The listing builds one solid part. Answer for the finished solid, in the listing's coordinates (mm). Face numbers are marked on the shaded views. Round coordinates to 2 decimals unless told otherwise and drop trailing zeros. Write each loop counter-clockwise with the first axis right and the second up, starting at its lowest first coordinate (ties: lowest second). Pieces come first, ordered by that corner, then holes. Notation, with made-up numbers: M -26,52.25 L 2,52.25 A21 ccw 2,83.25 Z; hole C 79.5,34.5 d3. An arc over 180 degrees is marked long. Write each question's results on one line, items separated by ' | '.
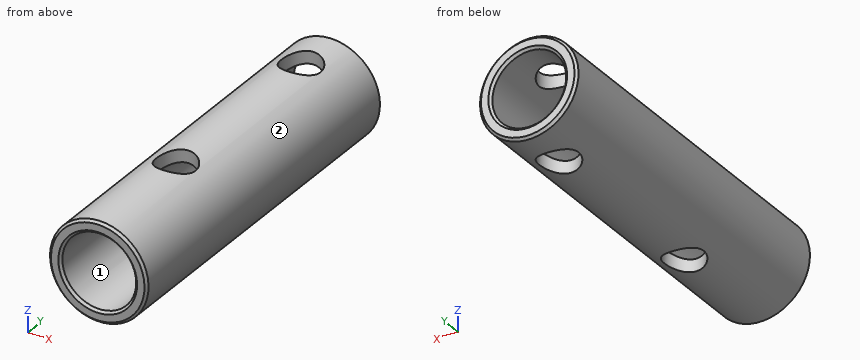
from build123d import *

# Parameters (mm, degrees)
SKIZZE1_R                       = 4
SKIZZE1_R_2                     = 3
AUFSATZ_LINEAR_AUSTRAGEN1_DEPTH = 30
FASE1_SIZE                      = 0.2
SKIZZE2_R                       = 1.6
SCHNITT_LINEAR_AUSTRAGEN1_DEPTH = 6


with BuildPart() as part:
    # Skizze1 → Aufsatz-Linear austragen1 (new body)
    with BuildSketch(Plane(origin=(0, 0, 0), x_dir=(1, 0, 0), z_dir=(0, 1, 0))):
        with Locations(Location((0, 0, 0), (0, 0, 270))):
            Circle(SKIZZE1_R)
        with Locations(Location((0, 0, 0), (0, 0, 270))):
            Circle(SKIZZE1_R_2, mode=Mode.SUBTRACT)
    extrude(amount=AUFSATZ_LINEAR_AUSTRAGEN1_DEPTH)

    # Fase1
    fase1_edges = [part.edges().sort_by_distance(p)[0] for p in [
        (0, 0, -4),
        (0, 30, -4),
        (0, 0, -3),
        (0, 30, -3),
    ]]
    chamfer(fase1_edges, length=FASE1_SIZE)

    # Skizze2 → Schnitt-Linear austragen1 (cut, symmetric)
    with BuildSketch(Plane.XY):
        with Locations((0, 26)):
            Circle(SKIZZE2_R)
        with Locations((0, 10)):
            Circle(SKIZZE2_R)
    extrude(amount=SCHNITT_LINEAR_AUSTRAGEN1_DEPTH, both=True, mode=Mode.SUBTRACT)


solid = part.part
1) The mould has two halves that part along X. Classify the marked faces 1 and 2: +X half, -X half, draft (parallel to the pull), parting line (faces both ways), or undercut.
Return value:
face 1: undercut | face 2: parting line
2) Each of these flat-tipped pins is pushed along its axis until it touches: pin 1 (1.5 mm diameter, centred on y = 12, z = 3, fed in from -X); pin 2 (1.5 mm diameter, centred on y = 23, z = 2, fed in from +X); pin 3 (1.5 mm diameter, centred on x = 2, y = 16, fed in from +Z); pin 4 (3 mm diameter, centred on x = -0.5, z = 0, fed in from -Y). Where does it stop, or does it pass through?
Return value:
pin 1: x = -3.31 | pin 2: x = 3.8 | pin 3: z = 3.8 | pin 4: through
3) Section D-D (y = 6.5) is taken. Determine the outline of the cut face in (x, z).
Return value:
outline: C 0,0 d8; hole C 0,0 d6
4) Section B-B (x = 0) is taken. State how many separate pieces and enclosed holes the cut face has, then the cut area to 3 significant figures.
Return value:
separate pieces: 6 | enclosed holes: 0 | area: 47.0 mm²
5) Find the intervals of material crossed by line 1 (X direction, y = 21.25, z = 0); line 2 (Y direction, x = 1.25, z = 3.5); line 3 (X direction, y = 22.5, z = 1.25), in increasing order.
Return value:
line 1: -4 to -3, 3 to 4 | line 2: 0 to 9, 11 to 25, 27 to 30 | line 3: -3.8 to -2.73, 2.73 to 3.8
6) Section C-C (y = 10) is taken. Determine the outline of the cut face in (x, z).
Return value:
outline: M -1.6,-3.67 L -1.6,-2.54 A3 cw -1.6,2.54 L -1.6,3.67 A4 ccw Z; M 1.6,-3.67 A4 ccw 1.6,3.67 L 1.6,2.54 A3 cw 1.6,-2.54 Z
7) Section A-A (z = 0) is taken. Determine the outline of the cut face in (x, y).
Return value:
outline: M -4,0.2 L -3.8,0 L -3.2,0 L -3,0.2 L -3,29.8 L -3.2,30 L -3.8,30 L -4,29.8 Z; M 3,0.2 L 3.2,0 L 3.8,0 L 4,0.2 L 4,29.8 L 3.8,30 L 3.2,30 L 3,29.8 Z
